Verification items for this drawing (mm, ordinates from the low corner). A direction names the side the tool comes from. Coordinates: 2 decimals unless noted, no trailing zeros. Order: outer loops, then holes, each group sorted by start corner. A loop starts at its lowest first (then second) coordinate and runs counter-clockwise, first axis right, second up.
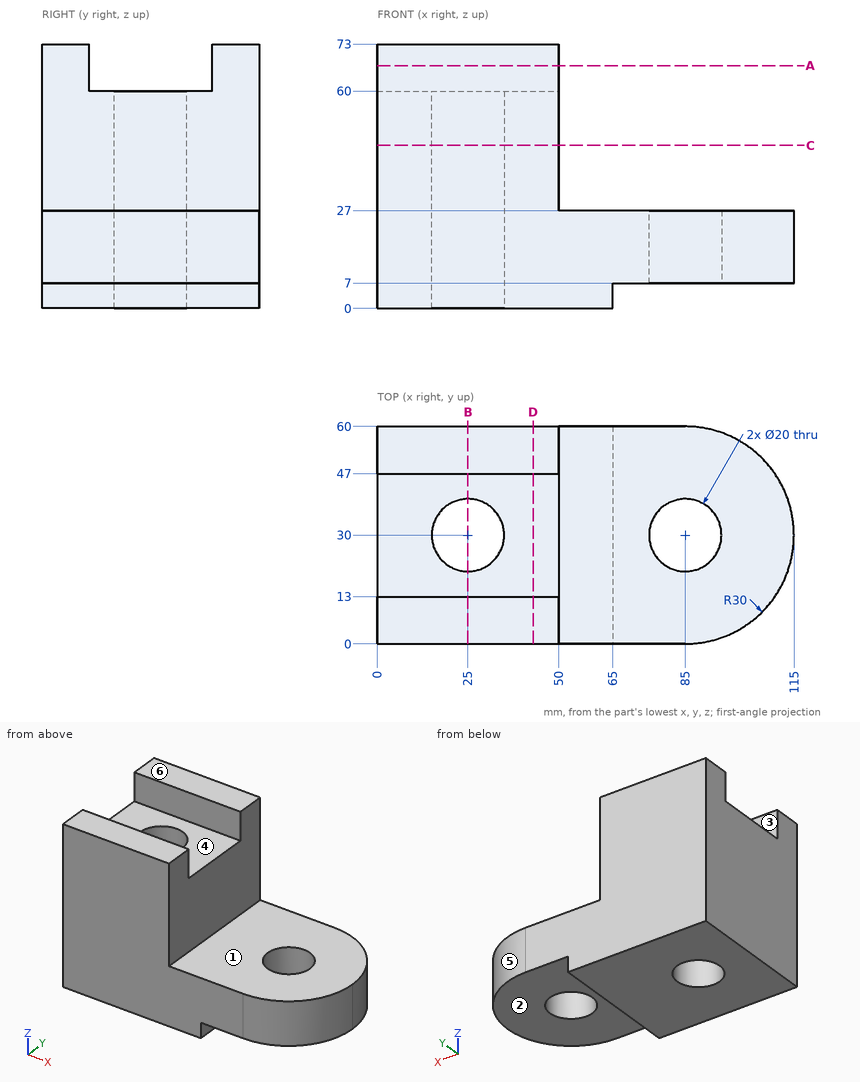
(1) Cross-section at A-A (z = 67). Enter the section's corners in (x, y).
Filled in:
outline: (0, 0) - (50, 0) - (50, 13) - (0, 13) - close; (0, 47) - (50, 47) - (50, 60) - (0, 60) - close
(2) Tool access check on the marked faces 1, 2 and 3. Record the directions out of +Z, -Z, +X, -X, +Y, -Y that give a thin tool (end or side, any length) a straight path to the whole face; none if there is none.
Filled in:
face 1: +Z, +X, +Y, -Y
face 2: -Z, +X, +Y, -Y
face 3: +Z, +X, -X
(3) Cross-section at B-B (x = 25). Enter the section's corners in (y, z), and give its area (3 significant figures).
Filled in:
outline: (0, 0) - (20, 0) - (20, 60) - (13, 60) - (13, 73) - (0, 73) - close; (40, 0) - (60, 0) - (60, 73) - (47, 73) - (47, 60) - (40, 60) - close
area: 2,740 mm2
(4) Cross-section at C-C (z = 45). Enter the section's corners in (x, y).
Filled in:
outline: (0, 0) - (50, 0) - (50, 60) - (0, 60) - close; hole circle Ø20 at (25, 30)
(5) Release check for a two-part mould opening along Y. For the marked faces 4, 5 and 6 record: +Y half, -Y half, draft (parallel to the pull), parting line (faces both ways), or undercut.
Filled in:
face 4: undercut
face 5: +Y half
face 6: draft
(6) Cross-section at D-D (x = 43). Enter the section's corners in (y, z), and give its area (3 significant figures).
Filled in:
outline: (0, 0) - (60, 0) - (60, 73) - (47, 73) - (47, 60) - (13, 60) - (13, 73) - (0, 73) - close
area: 3,940 mm2
(7) Go/stop test with flat-tipped pins: P1, Ø25, axis at x = 81.5, y = 20.5, coming from the -Z side; P2, Ø10, axis at x = 52, y = 11, coming from the -Z side; P3, Ø10, axis at y = 50.5, z = 24.5, coming from the +X side; P4, Ø23, axis at y = 28, z = 39, coming from the +X side. Record where each tip stops, or that it passes through.
Filled in:
P1: stops at z = 7
P2: stops at z = 0
P3: stops at x = 110.69
P4: stops at x = 50
(8) Thickness scan on probe 1 along Y at (x, z) = (25, 35.5); probe 2 along X at (y, z) = (21.5, 20.5); probe 3 along Z at (x, y) = (104.5, 24). Record the ranges inside material, lowest first.
Filled in:
probe 1: y = 0 to 20, 40 to 60
probe 2: x = 0 to 19.73, 30.27 to 79.73, 90.27 to 113.77
probe 3: z = 7 to 27
